The listing builds one solid part. Answer for the finished solid, in the listing's coordinates (mm). Face numbers are marked on the shaded views. A direction names the side the tool comes from. Give positions to 0.01 mm unless a question says otherwise; leave off trailing zeros. Write each loop counter-clockwise with the first axis right and the second up, starting at its lowest first coordinate (ties: lowest second). Pieces come first, ordered by that corner, then holes. Notation, with made-up numbers: (71, 48) - (104, 48) arc R9 ccw to (104, 53) - close; hole circle Ø2 at (-17.5, 74.5). An arc over 180 degrees is marked (long way). One line per item, written item: value. Start each with the question number.
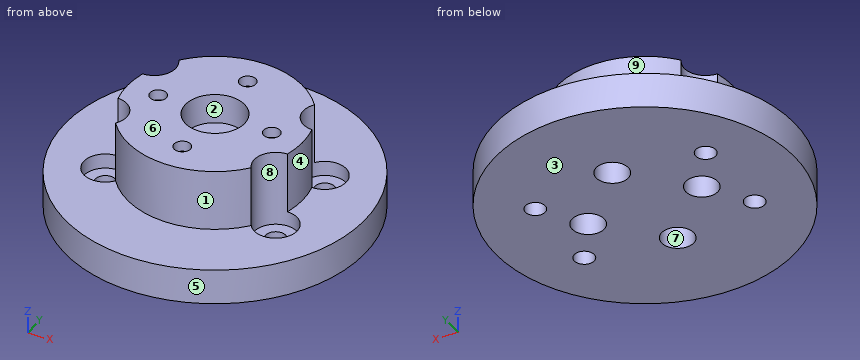
Autodesk Fusion 360 part; units mm, degrees
sketch "スケッチ1" plane through (0, 0, 0) normal (0, 0, 1) x (1, 0, 0)
  circle A0 centre (0, 0) radius 21
  dimension "d1" = 42
extrude "押し出し1" add sketch "スケッチ1" along normal blind 5
sketch "スケッチ2" plane through (0, 0, 5) normal (0, 0, 1) x (-1, 0, 0)
  circle A0 centre (0, 0) radius 21
  circle A1 centre (0, 0) radius 12.3
  dimension "d4" = 24.6
extrude "押し出し2" add sketch "スケッチ2" along normal blind 8.6 contours A1
sketch "スケッチ3" plane through (0, 0, 13.6) normal (0, 0, 1) x (-1, 0, 0)
  circle A0 centre (0, 0) radius 12.3
  circle A1 centre (0, 0) radius 4.15
  dimension "d7" = 8.3
extrude "押し出し3" cut sketch "スケッチ3" against normal blind 4.2 contours A1
sketch "スケッチ4" plane through (0, 0, 0) normal (0, 0, -1) x (1, 0, 0)
  circle A0 centre (0, 0) radius 21
  circle A1 centre (0, 0) radius 8
  circle A2 centre (0, -8) radius 1.15
  circle A3 centre (8, 0) radius 1.15
  circle A4 centre (0, 8) radius 1.15
  circle A5 centre (-8, 0) radius 1.15
  dimension "d10" = 16
  dimension "d11" = 2.3
  dimension "d12" = 2.3
  dimension "d13" = 2.3
  dimension "d14" = 2.3
extrude "押し出し4" cut sketch "スケッチ4" against normal through all contours A1 A3 | A1 A3 | A1 A4 | A1 A4 | A1 A2 | A1 A2 | A1 A5 | A1 A5
sketch "スケッチ5" plane through (0, 0, 0) normal (0, 0, -1) x (1, 0, 0)
  circle A0 centre (8, 0) radius 1.15
  circle A1 centre (0, 8) radius 1.15
  circle A2 centre (0, -8) radius 1.15
  circle A3 centre (-8, 0) radius 1.15
  circle A4 centre (0, 0) radius 21
  line L0 (12, -6) -> (-12, -6)
  line L1 (-12, -6) -> (-12, 6)
  line L2 (-12, 6) -> (12, 6)
  line L3 (12, 6) -> (12, -6)
  circle A5 centre (12, -6) radius 1.4
  circle A6 centre (-12, -6) radius 1.4
  circle A7 centre (12, 6) radius 1.4
  circle A8 centre (-12, 6) radius 1.4
  dimension "d16" = 24
  dimension "d17" = 12
  dimension "d18" = 12
  dimension "d19" = 6
  dimension "d20" = 2.8
  dimension "d21" = 2.8
  dimension "d22" = 2.8
  dimension "d23" = 2.8
extrude "押し出し5" cut sketch "スケッチ5" against normal through all contours L0 L1 A6 | L0 L1 A6 | L0 L3 A5 | L0 L3 A5 | L1 L2 A8 | L1 L2 A8 | L2 L3 A7 | L2 L3 A7
sketch "スケッチ6" plane through (0, 0, 0) normal (0, 0, -1) x (1, 0, 0)
  circle A0 centre (0, 0) radius 21
  circle A1 centre (-8, 0) radius 1.15
  circle A2 centre (0, -8) radius 1.15
  circle A3 centre (0, 8) radius 1.15
  circle A4 centre (8, 0) radius 1.15
  circle A5 centre (-12, 6) radius 1.4
  circle A6 centre (12, -6) radius 1.4
  circle A7 centre (-12, -6) radius 1.4
  circle A8 centre (12, 6) radius 1.4
  circle A9 centre (-8, 0) radius 2.25
  circle A10 centre (0, 8) radius 2.25
  circle A11 centre (8, 0) radius 2.25
  circle A12 centre (0, -8) radius 2.25
  dimension "d25" = 4.5
  dimension "d26" = 4.5
  dimension "d27" = 4.5
  dimension "d28" = 4.5
extrude "押し出し6" cut sketch "スケッチ6" against normal blind 12.1 contours A9 | A10 | A11 | A12
sketch "スケッチ7" plane through (0, 0, 13.6) normal (0, 0, 1) x (-1, 0, 0)
  circle A0 centre (12, -6) radius 3
  circle A1 centre (12, 6) radius 3
  circle A2 centre (-12, -6) radius 3
  circle A3 centre (-12, 6) radius 3
  dimension "d31" = 6
  dimension "d32" = 6
  dimension "d33" = 6
  dimension "d34" = 6
extrude "押し出し7" cut sketch "スケッチ7" against normal blind 10.7
equation "d18 = d16 / 2"
equation "d19 = d17 / 2"
Item 1: Straight lines are drawn through the part: line 1 along X through (y, z) = (0, 7.5); line 2 along X through (y, z) = (-6, 1.95); line 3 along Y through (x, z) = (-12, 4.5). For each, find the intervals that lie inside material, in ascending order.
Item 2: Find section A-A on y = 0. Determine the outline of the cut face in (x, z), plus the area to 3 significant figures.
Item 3: Find section C-C on z = 1. Give the number of separate pieces and of enclosed holes in the cut face, plus the area to 3 significant figures.
Item 4: The mould has two halves that part along X. Classify the marked faces 1, 2, 3 and 4: +X half, -X half, draft (parallel to the pull), parting line (faces both ways), or undercut.
Item 5: For the marked faces 5, 6, 7, 8 and 9, determine the directions among +Z, -Z, +X, -X, +Y, -Y from which every point of the face is accessible in a straight line to the end or side of a thin tool.
Item 6: Find section D-D on z = 10. Determine the outline of the cut face in (x, y).
Item 7: Each of these flat-tipped pins is pushed along its axis until it touches: pin 1 Ø3 at (y, z) = (-12, 11) entering from +X; pin 2 Ø1.5 at (y, z) = (-8, 9) entering from +X; pin 3 Ø1.3 at (x, y) = (8.5, -1) entering from -Z. Where does it stop, or does it pass through?
Values:
1. line 1: -12.3 to -10.25, -5.75 to 5.75, 10.25 to 12.3
1. line 2: -20.12 to -13.4, -10.6 to -1.03, 1.03 to 10.6, 13.4 to 20.12
1. line 3: -17.23 to -9, -3 to 3, 9 to 17.23
2. outline: (-21, 0) - (-10.25, 0) - (-10.25, 12.1) - (-9.15, 12.1) - (-9.15, 13.6) - (-12.3, 13.6) - (-12.3, 5) - (-21, 5) - close; (-6.85, 12.1) - (-5.75, 12.1) - (-5.75, 0) - (5.75, 0) - (5.75, 12.1) - (6.85, 12.1) - (6.85, 13.6) - (4.15, 13.6) - (4.15, 9.4) - (-4.15, 9.4) - (-4.15, 13.6) - (-6.85, 13.6) - close; (9.15, 12.1) - (10.25, 12.1) - (10.25, 0) - (21, 0) - (21, 5) - (12.3, 5) - (12.3, 13.6) - (9.15, 13.6) - close
2. area: 271 mm^2
3. separate pieces: 1
3. enclosed holes: 8
3. area: 1,300 mm^2
4. face 1: parting line
4. face 2: undercut
4. face 3: draft
4. face 4: +X half
5. face 5: +Z, -Z
5. face 6: +Z, +X, -X, +Y, -Y
5. face 7: -Z
5. face 8: +Z
5. face 9: +Z, +Y
6. outline: (-11.93, -3) arc R3 cw to (-9.56, -7.74) arc R12.3 ccw to (9.56, -7.74) arc R3 cw to (11.93, -3) arc R12.3 ccw to (11.93, 3) arc R3 cw to (9.56, 7.74) arc R12.3 ccw to (-9.56, 7.74) arc R3 cw to (-11.93, 3) arc R12.3 ccw to start; hole circle Ø4.5 at (-8, 0); hole circle Ø8.3 at (0, 0); hole circle Ø4.5 at (0, -8); hole circle Ø4.5 at (0, 8); hole circle Ø4.5 at (8, 0)
7. pin 1: x = 6.41
7. pin 2: x = 9.56
7. pin 3: z = 12.1
